Source: CAD feature listing. Evaluate the final solid. Frame: model axes, mm. A direction names the side the tool comes from. Round coordinates to 2 decimals unless told otherwise and drop trailing zeros. Write each loop counter-clockwise with the first axis right and the second up, starting at its lowest first coordinate (ties: lowest second). Pieces come first, ordered by that corner, then holes.
from build123d import *

# Parameters (mm, degrees)
SKETCH1_W           = 27
SKETCH1_H           = 27
BOSS_EXTRUDE1_DEPTH = 2
SKETCH2_W           = 27
SKETCH2_H           = 4
BOSS_EXTRUDE2_DEPTH = 8
SKETCH3_W           = 27
SKETCH3_H           = 7
BOSS_EXTRUDE3_DEPTH = 2
CHAMFER1_SIZE       = 1.5


with BuildPart() as part:
    # Sketch1 → Boss-Extrude1 (new body)
    with BuildSketch(Plane(origin=(0, 0, 0), x_dir=(1, 0, 0), z_dir=(0, 1, 0))):
        Rectangle(SKETCH1_W, SKETCH1_H)
    extrude(amount=BOSS_EXTRUDE1_DEPTH)

    # Sketch2 → Boss-Extrude2 (add)
    with BuildSketch(Plane.XZ):
        with Locations((0, -1.5)):
            Rectangle(SKETCH2_W, SKETCH2_H)
    extrude(amount=BOSS_EXTRUDE2_DEPTH)

    # Sketch3 → Boss-Extrude3 (add)
    with BuildSketch(Plane.XZ.offset(8)):
        with Locations((0, -1.5)):
            Rectangle(SKETCH3_W, SKETCH3_H)
    extrude(amount=-BOSS_EXTRUDE3_DEPTH)

    # Chamfer1
    chamfer1_edges = [part.edges().sort_by_distance(p)[0] for p in [
        (0, -6, -3.5),
        (0, -6, 0.5),
    ]]
    chamfer(chamfer1_edges, length=CHAMFER1_SIZE - 0.0001)  # a hair under: the kernel refuses the full size


solid = part.part
1) Section query B-B on y = -1.5. Return the cut outline in (x, z).
Taken from the geometry:
outline: (-13.5, -3.5) - (13.5, -3.5) - (13.5, 0.5) - (-13.5, 0.5) - close
2) Material intervals for line 1 (Y direction, x = 0.75, z = -5.25); line 2 (Y direction, x = -7.75, z = 0.75); line 3 (Z direction, x = 6.5, y = -6.25), sorted ascending.
Taken from the geometry:
line 1: y = 0 to 2
line 2: y = -8 to -4.75, 0 to 2
line 3: z = -5 to 2
3) Pull-direction query (Y, two-part tool) for faces 1 (the face through (0, -7, -5)), 2 (the face through (0, -5, 1)), 3 (the face through (0, -8, -1)); classes: released by +Y, released by -Y, zero draft, split by the parting line, or undercut.
Taken from the geometry:
face 1: zero draft
face 2: undercut
face 3: released by -Y
4) Section query C-C on z = 5.5. Return the cut outline in (x, y), then the cut area to 3 significant figures.
Taken from the geometry:
outline: (-13.5, 0) - (13.5, 0) - (13.5, 2) - (-13.5, 2) - close
area: 54.0 mm2
5) Reachability of faces 4 (the face through (0, -2, -3.5)), 5 (the face through (0, -2, 0.5)), 6 (the face through (0, -7, 2)) from +Z, -Z, +X, -X, +Y, -Y: full face, straight path, thin tool, end or side. Return the list, or none.
Taken from the geometry:
face 4: -Z, +X, -X
face 5: +Z, +X, -X
face 6: +Z, +X, -X, -Y
6) Contact query for flat-ended pins moving along their axis: P1, Ø1, axis at x = -7, y = -3.5, coming from the -Z side; P2, Ø5, axis at x = 1.5, z = -9.5, coming from the -Y side; P3, Ø2, axis at x = -6.5, y = -2, coming from the +Z side; P4, Ø5, axis at x = 0.5, y = -2, coming from the +Z side. Output: stop coordinate, or through.
Taken from the geometry:
P1: stops at z = -3.5
P2: stops at y = 0
P3: stops at z = 0.5
P4: stops at z = 13.5
